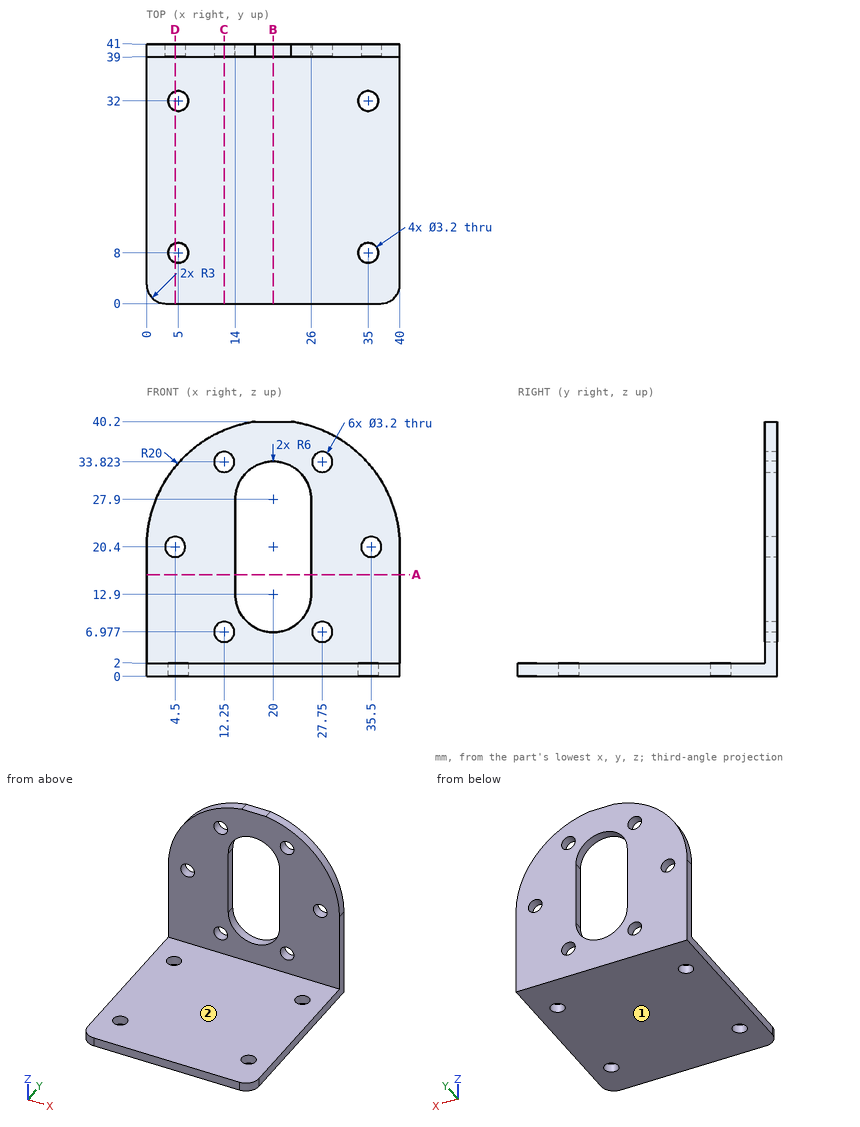
Verification items for this drawing (mm, ordinates from the low corner). A direction names the side the tool comes from. Round coordinates to 2 decimals unless told otherwise and drop trailing zeros. Loops run counter-clockwise (first coordinate to the right, second up) from the corner with the lowest first, then second, coordinate; pieces in that order, holes last. Notation, with made-up numbers: (51, 0.25) - (95, 0.25) arc R30 cw to (95, 37.25) - close; hole circle Ø8 at (30, 8). An arc over 180 degrees is marked (long way). Write item = value, one per line.
Q1. Material ranges on L1, parallel to Y at x = 5, z = 1; L2, parallel to X at y = 32, z = 0.4; L3, parallel to Y at x = 30.5, z = 9.5, recorded low to high.
Here are the results:
L1 = 0 to 6.4, 9.6 to 30.4, 33.6 to 41
L2 = 0 to 3.4, 6.6 to 33.4, 36.6 to 40
L3 = 39 to 41
Q2. Sectioned sample at A-A on z = 16. Record the boundary of the cut face in (x, y).
Here are the results:
outline = (0, 39) - (14, 39) - (14, 41) - (0, 41) - close; (26, 39) - (40, 39) - (40, 41) - (26, 41) - close
Q3. Sectioned sample at B-B on x = 20. Record the boundary of the cut face in (y, z), plus the area to 3 significant figures.
Here are the results:
outline = (0, 0) - (41, 0) - (41, 6.9) - (39, 6.9) - (39, 2) - (0, 2) - close; (39, 33.9) - (41, 33.9) - (41, 40.2) - (39, 40.2) - close
area = 104 mm^2
Q4. Sectioned sample at C-C on x = 12.25. Record the boundary of the cut face in (y, z).
Here are the results:
outline = (0, 0) - (41, 0) - (41, 5.38) - (39, 5.38) - (39, 2) - (0, 2) - close; (39, 8.58) - (41, 8.58) - (41, 32.22) - (39, 32.22) - close; (39, 35.42) - (41, 35.42) - (41, 38.84) - (39, 38.84) - close
Q5. Tool access check on the marked faces 1 and 2. Record the directions out of +Z, -Z, +X, -X, +Y, -Y that give a thin tool (end or side, any length) a straight path to the whole face; none if there is none.
Here are the results:
face_1 = -Z, +X, -X, +Y, -Y
face_2 = +Z, +X, -X, -Y
Q6. Sectioned sample at D-D on x = 4.5. Record the boundary of the cut face in (y, z).
Here are the results:
outline = (0, 0) - (6.48, 0) - (6.48, 2) - (0, 2) - close; (9.52, 0) - (30.48, 0) - (30.48, 2) - (9.52, 2) - close; (33.52, 0) - (41, 0) - (41, 18.8) - (39, 18.8) - (39, 2) - (33.52, 2) - close; (39, 22) - (41, 22) - (41, 33.04) - (39, 33.04) - close
Q7. Depth check by flat-ended pin: pin 1 (1 mm diameter, centred on x = 18, y = 9, fed in from -Z); pin 2 (12 mm diameter, centred on x = 33, y = 7, fed in from +Z); pin 3 (3.5 mm diameter, centred on x = 12.25, z = 33.82, fed in from -Y); pin 4 (1 mm diameter, centred on y = 40.5, z = 22, fed in from -X). Enter the tip coordinate at first touch or a pass-through.
Here are the results:
pin_1 = 0
pin_2 = 2
pin_3 = 39
pin_4 = 0.03
